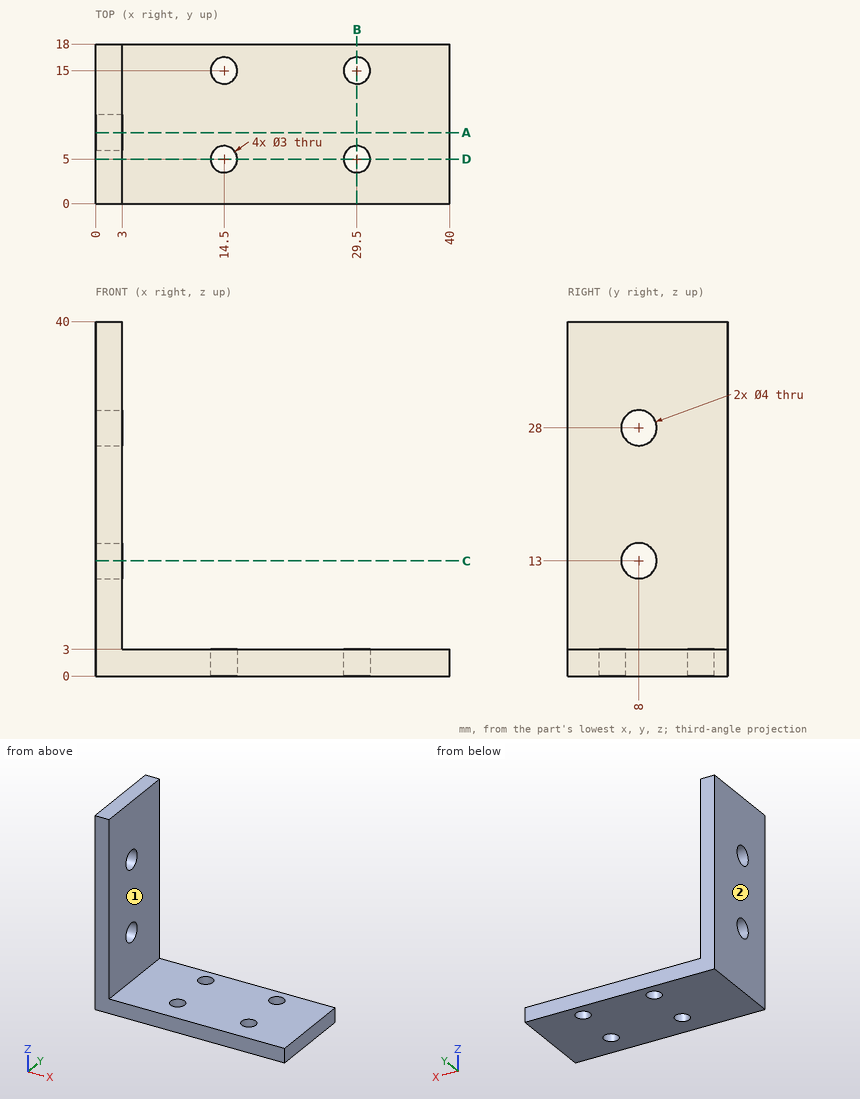
Geometry check sheet. Reference: drawing and pictorial views, mm from the part's lowest x, y, z. A direction names the side the tool comes from. Coordinates: 2 decimals unless noted, no trailing zeros. Write each loop counter-clockwise with the first axis right and the second up, starting at its lowest first coordinate (ties: lowest second). Pieces come first, ordered by that corner, then holes. Notation, with made-up numbers: M 19,57 L 78,57 A13 cw 78,68 Z; hole C 59,26.5 d5. An arc over 180 degrees is marked long. Use one line per item in the form item = value.
Item 1: Gauge pin test, flat ends, axial feed: pin 1 Ø3 at (y, z) = (3, 27.5) entering from +X; pin 2 Ø10 at (x, y) = (11, 7.5) entering from +Z. Record the tip position at first contact, or that the pin passes through.
Answer below:
pin_1 = 3
pin_2 = 3
Item 2: Sectioned sample at D-D, the plane y = 5. Record the cut outline in (x, z).
Answer below:
outline = M 0,0 L 13,0 L 13,3 L 3,3 L 3,40 L 0,40 Z; M 16,0 L 28,0 L 28,3 L 16,3 Z; M 31,0 L 40,0 L 40,3 L 31,3 Z
Item 3: Sectioned sample at A-A, the plane y = 8. Record the cut outline in (x, z).
Answer below:
outline = M 0,0 L 40,0 L 40,3 L 3,3 L 3,11 L 0,11 Z; M 0,15 L 3,15 L 3,26 L 0,26 Z; M 0,30 L 3,30 L 3,40 L 0,40 Z
Item 4: Set-up check for the marked faces 1 and 2: record each of +Z, -Z, +X, -X, +Y, -Y from which the full face is reachable in a straight line by a thin tool's end or side.
Answer below:
face_1 = +Z, +X, +Y, -Y
face_2 = +Z, -Z, -X, +Y, -Y
Item 5: Sectioned sample at B-B, the plane x = 29.5. Record the cut outline in (y, z).
Answer below:
outline = M 0,0 L 3.5,0 L 3.5,3 L 0,3 Z; M 6.5,0 L 13.5,0 L 13.5,3 L 6.5,3 Z; M 16.5,0 L 18,0 L 18,3 L 16.5,3 Z
Item 6: Sectioned sample at C-C, the plane z = 13. Record the cut outline in (x, y).
Answer below:
outline = M 0,0 L 3,0 L 3,6 L 0,6 Z; M 0,10 L 3,10 L 3,18 L 0,18 Z
Item 7: Material ranges on L1, parallel to Z at x = 0.65, y = 8; L2, parallel to Y at x = 29, z = 2; L3, parallel to X at y = 7.75, z = 7.5, recorded low to high. Write a range as from..to.
Answer below:
L1 = 0..11, 15..26, 30..40
L2 = 0..3.59, 6.41..13.59, 16.41..18
L3 = 0..3
